Can you work these out from the model? Positions are in its coordinate system, mm. Give positions to 0.01 mm unless a question says otherwise; leave off trailing zeros. Write each loop counter-clockwise with the first axis right and the second up, starting at its lowest first coordinate (ties: lowest second). Pieces come first, ordered by that corner, then holes. Notation, with made-up numbers: (-7.5, 87.25) -> (45.5, 87.25) arc R27 cw to (45.5, 105.25) -> close; hole circle Ø2 at (47.25, 51). An arc over 180 degrees is marked (long way). Answer as CSV lines item,"result". Start each with the question number.
1. If we section it at A-A on y = -4.75: Count the separate pieces of the cut face and the enclosed holes in it, plus the area to 3 significant figures.
2. I'm going to push flat-ended pins straight in: P1, Ø5, axis at x = -124.46, z = -41.89, coming from the -Y side; P2, Ø2.5, axis at x = -124.46, z = 97.81, coming from the +Y side. Where does each tip first touch, or does it pass through?
3. I need wall thicknesses on line 1 (Z direction, x = -123.75, y = -5.75); line 2 (X direction, y = -1.25, z = 98); line 3 (Z direction, x = -123.5, y = -2.75). Which ranges of each line are inside material? Lowest first, please. Write a range as [from, to].
4. If we section it at B-B on x = -130.5: Write out the boundary of the cut face in (y, z), plus the area to 3 significant figures.
```python
from build123d import *

# Parameters (mm, degrees)
F0_W     = 25.4
F0_H     = 165.1
F1_DEPTH = 6.35
F2_R     = 2.159
F3_DEPTH = 25.4
F4_R     = 12.69999


# Not quite as in the source:
# - a fillet or chamfer is up to 0.001 mm smaller than in the source, because OpenCascade refuses the exact size


with BuildPart() as f1:
    # F0 (on Front) → F1 (new body)
    with BuildSketch(Plane.XZ):
        with Locations((-124.4640206625, 27.955437386)):
            Rectangle(F0_W, F0_H)
    extrude(amount=F1_DEPTH)

    # F2 (on face) → F3 (cut)
    with BuildSketch(Plane.XZ.offset(6.35)):
        with Locations((-124.4640206625, 97.805437386)):
            Circle(F2_R)
        with Locations((-124.4640206625, -41.894562614)):
            Circle(F2_R)
    extrude(amount=-F3_DEPTH, mode=Mode.SUBTRACT)

    # F4 (radius 12.7 in the source; OpenCascade refuses exactly that, so slightly less here)
    f4_edges = [f1.edges().sort_by_distance(p)[0] for p in [
        (-137.164021, -3.175, 110.505437),
        (-111.764021, -3.175, 110.505437),
        (-137.164021, -3.175, -54.594563),
        (-111.764021, -3.175, -54.594563),
    ]]
    fillet(f4_edges, radius=F4_R)


solid = f1.part
```
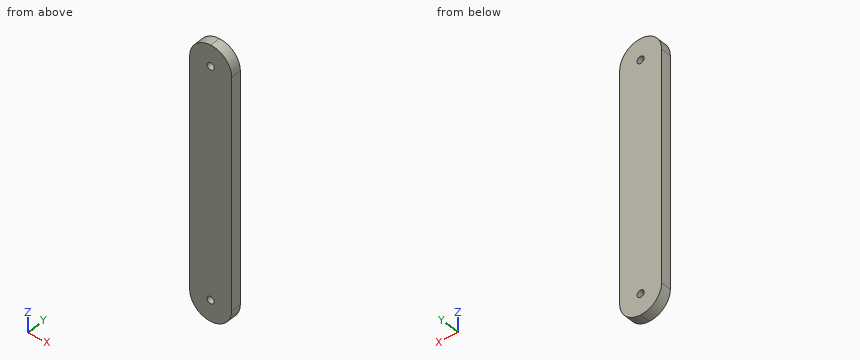
Computed values:
1,separate pieces,"1"
1,enclosed holes,"2"
1,area,"4,030 mm2"
2,P1,"stops at y = -6.35"
2,P2,"passes through"
3,line 1,"z = [-54.57, -43.93], [-39.86, 95.77], [99.84, 110.49]"
3,line 2,"x = [-137.16, -126.61], [-122.31, -111.77]"
3,line 3,"z = [-54.56, -43.83], [-39.96, 95.87], [99.74, 110.47]"
4,outline,"(-6.35, -53.07) -> (0, -53.07) -> (0, 108.98) -> (-6.35, 108.98) -> close"
4,area,"1,030 mm2"
